from build123d import *

# Parameters (mm, degrees)
BOSS_EXTRUDE1_DEPTH = 3
SKETCH2_R           = 8
CUT_EXTRUDE1_DEPTH  = 4
SKETCH5_R           = 72.5
CUT_EXTRUDE4_DEPTH  = 4
SKETCH4_R           = 80.5
SKETCH4_R_2         = 78.5
EXTRUDE_THIN1_DEPTH = 5
SKETCH6_R           = 1.5
BOSS_EXTRUDE2_DEPTH = 27
FILLET1_R           = 3
CUT_EXTRUDE5_DEPTH  = 10
FILLET2_R           = 20
SKETCH8_R           = 9.5
SKETCH8_R_2         = 8
EXTRUDE_THIN2_DEPTH = 2


with BuildPart() as part:
    # Sketch1 → Boss-Extrude1 (new body)
    with BuildSketch(Plane(origin=(0, 0, 0), x_dir=(1, 0, 0), z_dir=(0, 1, 0))):
        with BuildLine():
            Line((-115, -100), (115, -100))
            ThreePointArc((115, -100), (122.071067812, -97.071067812), (125, -90))
            Line((125, -90), (125, 90))
            ThreePointArc((125, 90), (122.071067812, 97.071067812), (115, 100))
            Line((115, 100), (-115, 100))
            ThreePointArc((-115, 100), (-122.071067812, 97.071067812), (-125, 90))
            Line((-125, 90), (-125, -90))
            ThreePointArc((-125, -90), (-122.071067812, -97.071067812), (-115, -100))
        make_face()
    extrude(amount=BOSS_EXTRUDE1_DEPTH)

    # Sketch2 → Cut-Extrude1 (cut, through all)
    with BuildSketch(Plane(origin=(0, 3, 0), x_dir=(1, 0, 0), z_dir=(0, 1, 0))):
        with Locations((-97.5, 0)):
            Circle(SKETCH2_R)
    cut_extrude1 = extrude(amount=-CUT_EXTRUDE1_DEPTH, mode=Mode.SUBTRACT)

    # Mirror1: Cut-Extrude1 across plane
    add(cut_extrude1.mirror(Plane(origin=(0, 0, 0), x_dir=(0, 0, 1), z_dir=(1, 0, 0))), mode=Mode.SUBTRACT)

    # Sketch5 → Cut-Extrude4 (cut, through all)
    with BuildSketch(Plane(origin=(0, 0, 0), x_dir=(1, 0, 0), z_dir=(0, 1, 0))):
        Circle(SKETCH5_R)
    extrude(amount=CUT_EXTRUDE4_DEPTH, mode=Mode.SUBTRACT)

    # Sketch4 → Extrude-Thin1 (add)
    with BuildSketch(Plane(origin=(0, 0, 0), x_dir=(1, 0, 0), z_dir=(0, 1, 0))):
        Circle(SKETCH4_R)
        Circle(SKETCH4_R_2, mode=Mode.SUBTRACT)
    extrude(amount=-EXTRUDE_THIN1_DEPTH)

    # Sketch6 → Boss-Extrude2 (add)
    with BuildSketch(Plane(origin=(0, 3, 0), x_dir=(1, 0, 0), z_dir=(0, 1, 0))):
        with BuildLine():
            ThreePointArc((-125, -17.5), (-124.121320344, -19.621320344), (-122, -20.5))
            Line((-122, -20.5), (-105.5, -20.5))
            ThreePointArc((-105.5, -20.5), (-103.378679656, -19.621320344), (-102.5, -17.5))
            Line((-102.5, -17.5), (-102.5, -9.797958971))
            ThreePointArc((-102.5, -9.797958971), (-108.5, 0), (-102.5, 9.797958971))
            Line((-102.5, 9.797958971), (-102.5, 17.5))
            ThreePointArc((-102.5, 17.5), (-103.378679656, 19.621320344), (-105.5, 20.5))
            Line((-105.5, 20.5), (-122, 20.5))
            ThreePointArc((-122, 20.5), (-124.121320344, 19.621320344), (-125, 17.5))
            Line((-125, 17.5), (-125, -17.5))
        make_face()
        with Locations((-105.5, -17.5)):
            Circle(SKETCH6_R, mode=Mode.SUBTRACT)
        with Locations((-105.5, 17.5)):
            Circle(SKETCH6_R, mode=Mode.SUBTRACT)
    extrude(amount=BOSS_EXTRUDE2_DEPTH)

    # Fillet1
    fillet1_edges = [part.edges().sort_by_distance(p)[0] for p in [
        (-102.5, 16.5, 9.797958971),
        (-102.5, 16.5, -9.797958971),
    ]]
    fillet(fillet1_edges, radius=FILLET1_R)

    # Sketch7 → Cut-Extrude5 (cut)
    with BuildSketch(Plane(origin=(0, 3, 0), x_dir=(1, 0, 0), z_dir=(0, 1, 0))):
        with BuildLine():
            Line((-125, 90), (-125, 30))
            Line((-125, 30), (-25, 100))
            Line((-25, 100), (-115, 100))
            ThreePointArc((-115, 100), (-122.071067812, 97.071067812), (-125, 90))
        make_face()
        with BuildLine():
            Line((25, 100), (125, 30))
            Line((125, 30), (125, 90))
            ThreePointArc((125, 90), (122.071067812, 97.071067812), (115, 100))
            Line((115, 100), (25, 100))
        make_face()
        with BuildLine():
            Line((125, -30), (25, -100))
            Line((25, -100), (115, -100))
            ThreePointArc((115, -100), (122.071067812, -97.071067812), (125, -90))
            Line((125, -90), (125, -30))
        make_face()
        with BuildLine():
            ThreePointArc((-125, -90), (-122.071067812, -97.071067812), (-115, -100))
            Line((-115, -100), (-25, -100))
            Line((-25, -100), (-125, -30))
            Line((-125, -30), (-125, -90))
        make_face()
    extrude(amount=-CUT_EXTRUDE5_DEPTH, mode=Mode.SUBTRACT)

    # Fillet2
    fillet2_edges = [part.edges().sort_by_distance(p)[0] for p in [
        (-125, 1.5, 30),
        (-25, 1.5, 100),
        (125, 1.5, 30),
        (25, 1.5, 100),
        (25, 1.5, -100),
        (125, 1.5, -30),
        (-125, 1.5, -30),
        (-25, 1.5, -100),
    ]]
    fillet(fillet2_edges, radius=FILLET2_R)

    # Sketch8 → Extrude-Thin2 (add)
    with BuildSketch(Plane(origin=(0, 3, 0), x_dir=(1, 0, 0), z_dir=(0, 1, 0))):
        with Locations((-97.5, 0)):
            Circle(SKETCH8_R)
        with Locations((-97.5, 0)):
            Circle(SKETCH8_R_2, mode=Mode.SUBTRACT)
        with Locations((97.5, 0)):
            Circle(SKETCH8_R)
        with Locations((97.5, 0)):
            Circle(SKETCH8_R_2, mode=Mode.SUBTRACT)
    extrude(amount=EXTRUDE_THIN2_DEPTH)


solid = part.part
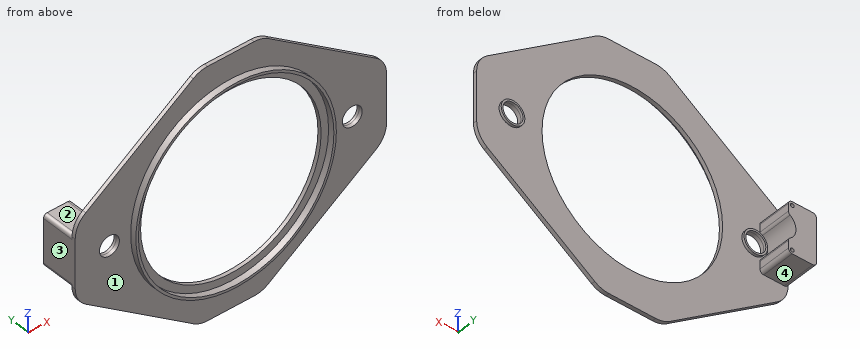
Check sheet for the modelled part. Datum: model origin and axes. Units: mm. Face numbers are marked on the shaded views. A direction names the side the tool comes from. Round coordinates to 2 decimals unless told otherwise and drop trailing zeros. Order: outer loops, then holes, each group sorted by start corner. A loop starts at its lowest first (then second) coordinate and runs counter-clockwise, first axis right, second up.
(1) Scan lines: probe 1 along X at (y, z) = (4, 0); probe 2 along X at (y, z) = (1.5, 0); probe 3 along Z at (x, y) = (-105.5, 22.5). Record each from-to range of solid material in increasing order.
(2) Cross-section at C-C, the plane y = 9. Enter the section's corners in (x, z), and give its area (3 significant figures).
(3) Access from +Z, -Z, +X, -X, +Y, -Y to the whole of each face (thin tool, end or side, straight path). Record for the marked faces 1, 2, 3 and 4.
(4) Cross-section at B-B, the plane z = 0. State how many separate pieces and enclosed holes the cut face has, and give its area (4 significant figures).
(5) Go/stop test with flat-tipped pins: P1, Ø3, axis at y = 21.5, z = -15.5, coming from the +X side; P2, Ø5, axis at x = -113.5, y = 14, coming from the +Z side; P3, Ø13, axis at x = 97.5, z = 0, coming from the +Y side; P4, Ø9.5, axis at x = -94, z = 1.5, coming from the +Y side. Record where each tip stops, or that it passes through.
(6) Cross-section at A-A, the plane x = -97.5. Enter the section's corners in (y, z).
(7) Cross-section at D-D, the plane z = -40.5. Enter the section's corners in (x, y), and give its area (3 significant figures).
Check sheet entries:
1. probe 1: x = -125 to -108.5, -107 to -105.5, -89.5 to -88, 88 to 89.5, 105.5 to 107
1. probe 2: x = -125 to -105.5, -89.5 to -72.5, 72.5 to 89.5, 105.5 to 125
1. probe 3: z = -20.5 to -19, -16 to -7.55, 7.55 to 16, 19 to 20.5
2. outline: (-125, -17.5) arc R3 ccw to (-122, -20.5) - (-105.5, -20.5) arc R3 ccw to (-102.5, -17.5) - (-102.5, -11.49) arc R3 ccw to (-103.79, -9.03) arc R11 cw to (-103.79, 9.03) arc R3 ccw to (-102.5, 11.49) - (-102.5, 17.5) arc R3 ccw to (-105.5, 20.5) - (-122, 20.5) arc R3 ccw to (-125, 17.5) - close; hole circle Ø3 at (-105.5, -17.5); hole circle Ø3 at (-105.5, 17.5)
2. area: 816 mm2
3. face 1: -Y
3. face 2: +Z, +X, -X, +Y
3. face 3: +Z, -Z, -X, +Y, -Y
3. face 4: -Z, +X, -X, +Y
4. separate pieces: 4
4. enclosed holes: 0
4. area: 696.5 mm2
5. P1: stops at x = -102.5
5. P2: stops at z = 20.5
5. P3: passes through
5. P4: stops at y = 5
6. outline: (0, -49.25) - (3, -49.25) - (3, -9.5) - (5, -9.5) - (5, -8) - (0, -8) - close; (0, 8) - (5, 8) - (5, 9.5) - (3, 9.5) - (3, 49.25) - (0, 49.25) - close
7. outline: (-110, 0) - (-69.57, 0) - (-69.57, -5) - (-67.25, -5) - (-67.25, 0) - (-60.13, 0) - (-60.13, 3) - (-110, 3) - close; (60.13, 0) - (67.25, 0) - (67.25, -5) - (69.57, -5) - (69.57, 0) - (110, 0) - (110, 3) - (60.13, 3) - close
7. area: 322 mm2
